Here's how the part is built. I have some questions about the finished solid (model axes, mm). A direction names the side the tool comes from. Give positions to 0.01 mm unless a question says otherwise; leave off trailing zeros. Write each loop counter-clockwise with the first axis right and the second up, starting at its lowest first coordinate (ties: lowest second). Pieces come first, ordered by that corner, then holes. Notation, with made-up numbers: (33, 42.25) -> (90, 42.25) arc R30 ccw to (90, 79.25) -> close; hole circle Ø9 at (6.5, 30.5). An arc over 180 degrees is marked (long way). Put each result on its own line as item: value. Start each with the question number.
from build123d import *

# Parameters (mm, degrees)
F0_W        = 50.8
F0_H        = 38.1
F1_DEPTH    = 12.7
F2_DEPTH    = 8.89
F3_W        = 10.16
F3_H        = 6.9189891219
F3_H_2      = 6.9088
F4_DEPTH    = 1.27
F5_T1_DEPTH = 18.6794189943
F5_T3_DEPTH = 15.4384081162
F6_T1_DEPTH = 15.4384081162
F6_T3_DEPTH = 18.6794189943
F6_T5_DEPTH = 18.6794189943
F6_T7_DEPTH = 18.6794189943
F6_T9_DEPTH = 15.4282189943


# Not quite as in the source:
# - a fillet or chamfer that OpenCascade refuses, or shapes differently, is made with other operations: its cross-section is extruded or revolved along the edge and cut away or added


with BuildPart() as f1:
    # F0 (on Top) → F1 (new body)
    with BuildSketch(Plane.XY):
        with BuildLine():
            Line((26.8096346408, 46.6933250427), (-49.3903653592, 46.6933250427))
            Line((-49.3903653592, 46.6933250427), (-49.3903653592, -52.5104318142))
            ThreePointArc((-49.3903653592, -52.5104318142), (-45.6706214803, -61.4906879353), (-36.6903653592, -65.2104318142))
            Line((-36.6903653592, -65.2104318142), (14.1096346408, -65.2104318142))
            ThreePointArc((14.1096346408, -65.2104318142), (23.0898907619, -61.4906879353), (26.8096346408, -52.5104318142))
            Line((26.8096346408, -52.5104318142), (26.8096346408, 46.6933250427))
        make_face()
        with BuildLine():
            Line((14.1096346408, 112.5895681858), (-36.6903653592, 112.5895681858))
            ThreePointArc((-36.6903653592, 112.5895681858), (-45.6706214803, 108.8698243069), (-49.3903653592, 99.8895681858))
            Line((-49.3903653592, 99.8895681858), (-49.3903653592, 46.6933250427))
            Line((-49.3903653592, 46.6933250427), (26.8096346408, 46.6933250427))
            Line((26.8096346408, 46.6933250427), (26.8096346408, 99.8895681858))
            ThreePointArc((26.8096346408, 99.8895681858), (23.0898907619, 108.8698243069), (14.1096346408, 112.5895681858))
        make_face()
        with Locations((-11.2903653592, 80.8395681858)):
            Rectangle(F0_W, F0_H, mode=Mode.SUBTRACT)
    extrude(amount=F1_DEPTH)

    # F0 (on Top) → F2 (join)
    with BuildSketch(Plane.XY):
        with Locations((-11.2903653592, 80.8395681858)):
            Rectangle(F0_W, F0_H)
    extrude(amount=F2_DEPTH)

    # F3 (on face) → F4 (join)
    with BuildSketch(Plane.XY.offset(12.7)):
        with Locations((-33.6411841828, 39.4687093794)):
            Rectangle(F3_W, F3_H)
        with Locations((-18.4011841828, 39.4687093794)):
            Rectangle(F3_W, F3_H)
        with Locations((-3.1611841828, 39.4738039404)):
            Rectangle(F3_W, F3_H_2)
        with Locations((14.2273069042, 39.4738039404)):
            Rectangle(F3_W, F3_H_2)
    extrude(amount=F4_DEPTH)

    # F5: fillet of radius 1.778 on 4 edges, made by hand

    # F5_s2 → F5_t1 (cut)
    with BuildSketch(Plane.YZ.offset(-42.9808936799)):
        with BuildLine():
            ThreePointArc((42.9282039404, 12.7), (42.2868783752, 13.6175714644), (41.2243201415, 13.97))
            Line((41.2243201415, 13.97), (42.9282039404, 13.97))
            Line((42.9282039404, 13.97), (42.9282039404, 12.7))
        make_face()
        with BuildLine():
            ThreePointArc((36.0092148185, 12.7), (36.6505403836, 13.6175714644), (37.7130986173, 13.97))
            Line((37.7130986173, 13.97), (36.0092148185, 13.97))
            Line((36.0092148185, 13.97), (36.0092148185, 12.7))
        make_face()
    extrude(amount=F5_T1_DEPTH, mode=Mode.SUBTRACT)

    # F5_s4 → F5_t3 (cut)
    with BuildSketch(Plane.XZ.offset(-47.1879134375)):
        with BuildLine():
            ThreePointArc((-38.7211841828, 12.7), (-38.0798586176, 13.6175714644), (-37.0173003839, 13.97))
            Line((-37.0173003839, 13.97), (-38.7211841828, 13.97))
            Line((-38.7211841828, 13.97), (-38.7211841828, 12.7))
        make_face()
        with BuildLine():
            ThreePointArc((-28.5611841828, 12.7), (-29.2025097479, 13.6175714644), (-30.2650679816, 13.97))
            Line((-30.2650679816, 13.97), (-28.5611841828, 13.97))
            Line((-28.5611841828, 13.97), (-28.5611841828, 12.7))
        make_face()
    extrude(amount=F5_T3_DEPTH, mode=Mode.SUBTRACT)

    # F6: fillet of radius 1.778 on 12 edges, made by hand

    # F6_s2 → F6_t1 (cut)
    with BuildSketch(Plane.XZ.offset(-47.1879134375)):
        with BuildLine():
            ThreePointArc((-23.4811841828, 12.7), (-22.8398586176, 13.6175714644), (-21.7773003839, 13.97))
            Line((-21.7773003839, 13.97), (-23.4811841828, 13.97))
            Line((-23.4811841828, 13.97), (-23.4811841828, 12.7))
        make_face()
        with BuildLine():
            ThreePointArc((-13.3211841828, 12.7), (-13.9625097479, 13.6175714644), (-15.0250679816, 13.97))
            Line((-15.0250679816, 13.97), (-13.3211841828, 13.97))
            Line((-13.3211841828, 13.97), (-13.3211841828, 12.7))
        make_face()
    extrude(amount=F6_T1_DEPTH, mode=Mode.SUBTRACT)

    # F6_s4 → F6_t3 (cut)
    with BuildSketch(Plane.YZ.offset(-27.7408936799)):
        with BuildLine():
            ThreePointArc((36.0092148185, 12.7), (36.6505403836, 13.6175714644), (37.7130986173, 13.97))
            Line((37.7130986173, 13.97), (36.0092148185, 13.97))
            Line((36.0092148185, 13.97), (36.0092148185, 12.7))
        make_face()
        with BuildLine():
            ThreePointArc((42.9282039404, 12.7), (42.2868783752, 13.6175714644), (41.2243201415, 13.97))
            Line((41.2243201415, 13.97), (42.9282039404, 13.97))
            Line((42.9282039404, 13.97), (42.9282039404, 12.7))
        make_face()
    extrude(amount=F6_T3_DEPTH, mode=Mode.SUBTRACT)

    # F6_s6 → F6_t5 (cut)
    with BuildSketch(Plane.YZ.offset(-12.5008936799)):
        with BuildLine():
            ThreePointArc((42.9282039404, 12.7), (42.2868783752, 13.6175714644), (41.2243201415, 13.97))
            Line((41.2243201415, 13.97), (42.9282039404, 13.97))
            Line((42.9282039404, 13.97), (42.9282039404, 12.7))
        make_face()
        with BuildLine():
            ThreePointArc((36.0194039404, 12.7), (36.6607295055, 13.6175714644), (37.7232877392, 13.97))
            Line((37.7232877392, 13.97), (36.0194039404, 13.97))
            Line((36.0194039404, 13.97), (36.0194039404, 12.7))
        make_face()
    extrude(amount=F6_T5_DEPTH, mode=Mode.SUBTRACT)

    # F6_s8 → F6_t7 (cut)
    with BuildSketch(Plane.YZ.offset(4.8875974071)):
        with BuildLine():
            ThreePointArc((42.9282039404, 12.7), (42.2868783752, 13.6175714644), (41.2243201415, 13.97))
            Line((41.2243201415, 13.97), (42.9282039404, 13.97))
            Line((42.9282039404, 13.97), (42.9282039404, 12.7))
        make_face()
        with BuildLine():
            ThreePointArc((36.0194039404, 12.7), (36.6607295055, 13.6175714644), (37.7232877392, 13.97))
            Line((37.7232877392, 13.97), (36.0194039404, 13.97))
            Line((36.0194039404, 13.97), (36.0194039404, 12.7))
        make_face()
    extrude(amount=F6_T7_DEPTH, mode=Mode.SUBTRACT)

    # F6_s10 → F6_t9 (cut)
    with BuildSketch(Plane.XZ.offset(-47.1879134375)):
        with BuildLine():
            ThreePointArc((9.1473069042, 12.7), (9.7886324694, 13.6175714644), (10.8511907031, 13.97))
            Line((10.8511907031, 13.97), (9.1473069042, 13.97))
            Line((9.1473069042, 13.97), (9.1473069042, 12.7))
        make_face()
        with BuildLine():
            ThreePointArc((19.3073069042, 12.7), (18.665981339, 13.6175714644), (17.6034231053, 13.97))
            Line((17.6034231053, 13.97), (19.3073069042, 13.97))
            Line((19.3073069042, 13.97), (19.3073069042, 12.7))
        make_face()
        with BuildLine():
            ThreePointArc((-8.2411841828, 12.7), (-7.5998586176, 13.6175714644), (-6.5373003839, 13.97))
            Line((-6.5373003839, 13.97), (-8.2411841828, 13.97))
            Line((-8.2411841828, 13.97), (-8.2411841828, 12.7))
        make_face()
        with BuildLine():
            ThreePointArc((1.9188158172, 12.7), (1.2774902521, 13.6175714644), (0.2149320184, 13.97))
            Line((0.2149320184, 13.97), (1.9188158172, 13.97))
            Line((1.9188158172, 13.97), (1.9188158172, 12.7))
        make_face()
    extrude(amount=F6_T9_DEPTH, mode=Mode.SUBTRACT)


solid = f1.part
1) I want a section at B-B, the plane y = 71.5. Write out the boundary of the cut face in (x, z), and give its area (3 significant figures).
2) I want a section at A-A, the plane z = 11. Write out the boundary of the cut face in (x, y), and give its area (3 significant figures).
3) Which directions (+Z, -Z, +X, -X, +Y, -Y) give clear straight access to the entire face, cutting with the end or side of a thin tool? Please do faces 4 (the flat face through (-36.69, 81, 11)), 5 (the cylindrical face through (23.19, 108.77, 6.26)).
4) I want a section at C-C, the plane y = -1. Write out the boundary of the cut face in (x, z), and give its area (3 significant figures).
5) I need wall thicknesses on probe 1 along Y at (x, z) = (-19, 12); probe 2 along X at (y, z) = (73, 10); probe 3 along Z at (x, y) = (12, 9). Which ranges of each line are inside material? Lowest first, please.
6) Thinking about a two-plate mould opening in Y: for faces 1 (the flat face through (14.11, 81, 11)), 2 (the flat face through (-34, 39, 13.97)), 3 (the cylindrical face through (-45.77, -61.39, 6.26)), which applies, released by +Y, released by -Y, zero draft, split by the parting line, or undercut?
Established:
1. outline: (-49.39, 0) -> (26.81, 0) -> (26.81, 12.7) -> (14.11, 12.7) -> (14.11, 8.89) -> (-36.69, 8.89) -> (-36.69, 12.7) -> (-49.39, 12.7) -> close
1. area: 774 mm2
2. outline: (-49.39, -52.51) arc R12.7 ccw to (-36.69, -65.21) -> (14.11, -65.21) arc R12.7 ccw to (26.81, -52.51) -> (26.81, 99.89) arc R12.7 ccw to (14.11, 112.59) -> (-36.69, 112.59) arc R12.7 ccw to (-49.39, 99.89) -> close; hole (-36.69, 61.79) -> (14.11, 61.79) -> (14.11, 99.89) -> (-36.69, 99.89) -> close
2. area: 11,500 mm2
3. face 4: +Z
3. face 5: +Z, -Z, +X, +Y
4. outline: (-49.39, 0) -> (26.81, 0) -> (26.81, 12.7) -> (-49.39, 12.7) -> close
4. area: 968 mm2
5. probe 1: y = -65.21 to 61.79, 99.89 to 112.59
5. probe 2: x = -49.39 to -36.69, 14.11 to 26.81
5. probe 3: z = 0 to 12.7
6. face 1: undercut
6. face 2: zero draft
6. face 3: released by -Y
